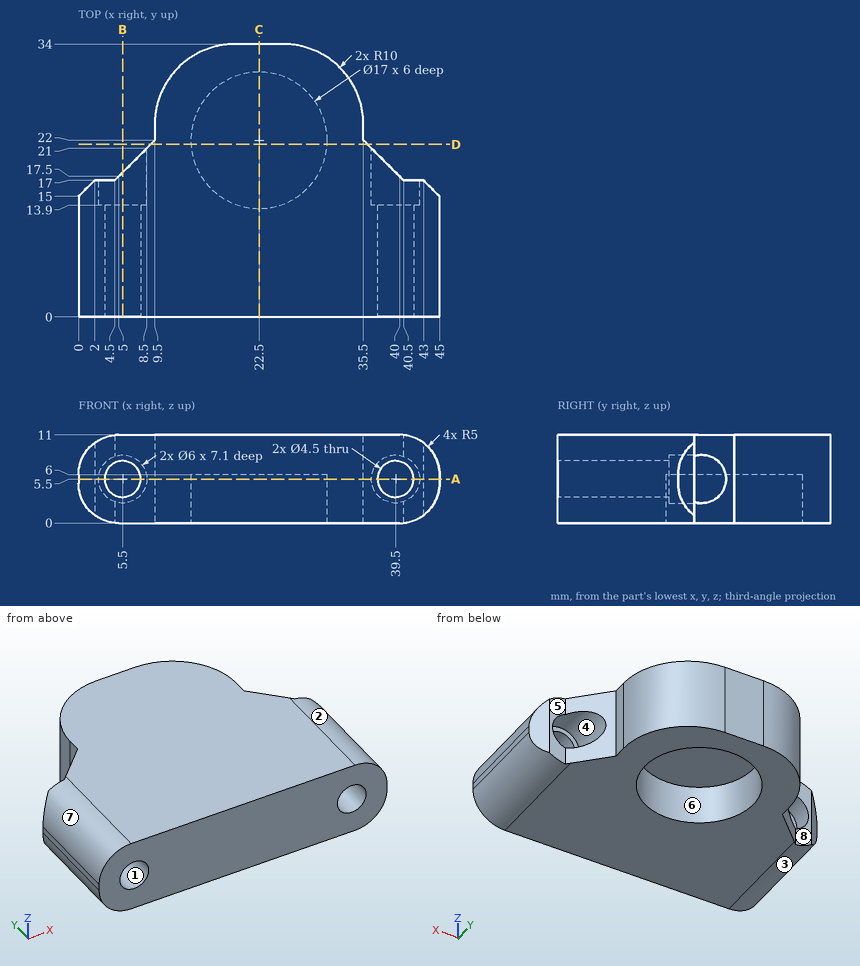
Study the drawing (mm; zero at the part's minimum x, y, z) and answer. A direction names the side the tool comes from. Give positions to 0.01 mm unless a question says otherwise; leave off trailing zeros. Write each loop counter-clockwise with the first axis right and the second up, starting at its lowest first coordinate (ties: lowest second). Pieces come first, ordered by that corner, then holes. Notation, with made-up numbers: (41, -25.75) -> (73, -25.75) arc R26 ccw to (73, 1.25) -> close; hole circle Ø11 at (4, -15). An arc over 180 degrees is marked (long way). Answer in a Markdown table with one row per item.
1) Section A-A on z = 5.5 is taken. Count the separate pieces of the cut face and the enclosed holes in it, plus the area to 3 significant figures.
Results list:
| item | result |
|---|---|
| separate pieces | 3 |
| enclosed holes | 1 |
| area | 780 mm^2 |
2) Each of these flat-tipped pins is pushed along its axis until it touches: pin 1 Ø5 at (x, y) = (26.5, 23) entering from -Z; pin 2 Ø5 at (x, z) = (39.5, 5.5) entering from -Y; pin 3 Ø0.8 at (x, z) = (41.5, 6.5) entering from +Y; pin 4 Ø3 at (x, z) = (40, 5.5) entering from +Y. Where does it stop, or does it pass through?
Results list:
| item | result |
|---|---|
| pin 1 | z = 6 |
| pin 2 | y = 0 |
| pin 3 | y = 13.9 |
| pin 4 | through |
3) Section C-C on x = 22.5 is taken. Give the vertices of the cut face in (y, z).
Results list:
| item | result |
|---|---|
| outline | (0, 0) -> (13.5, 0) -> (13.5, 6) -> (30.5, 6) -> (30.5, 0) -> (34, 0) -> (34, 11) -> (0, 11) -> close |
4) Section D-D on y = 21.5 is taken. Give the vertices of the cut face in (x, z).
Results list:
| item | result |
|---|---|
| outline | (9, 0) -> (14.01, 0) -> (14.01, 6) -> (30.99, 6) -> (30.99, 0) -> (36, 0) -> (36, 11) -> (9, 11) -> close |
5) Section B-B on x = 5.5 is taken. Give the vertices of the cut face in (y, z), plus the area to 3 significant figures.
Results list:
| item | result |
|---|---|
| outline | (0, 0) -> (18, 0) -> (18, 2.5) -> (13.9, 2.5) -> (13.9, 3.25) -> (0, 3.25) -> close; (0, 7.75) -> (13.9, 7.75) -> (13.9, 8.5) -> (18, 8.5) -> (18, 11) -> (0, 11) -> close |
| area | 111 mm^2 |
6) Determine the mould class of the marked faces 1, 2 and 3 for opening direction Z: released by +Z, released by -Z, zero draft, split by the parting line, or undercut.
Results list:
| item | result |
|---|---|
| face 1 | undercut |
| face 2 | released by +Z |
| face 3 | released by -Z |
7) Straight lines are drawn through the part: line 1 (Z direction, x = 39.5, y = 9); line 2 (Y direction, x = 22.5, z = 3.25); line 3 (X direction, y = 7, z = 4). For each, find the intervals that lie inside material, in ascending order. Write a range as [from, to].
Results list:
| item | result |
|---|---|
| line 1 | [0, 3.25], [7.75, 11] |
| line 2 | [0, 13.5], [30.5, 34] |
| line 3 | [0.1, 3.82], [7.18, 37.82], [41.18, 44.9] |
8) A tool of negligible diameter and unlimited length cuts with its end or side. For the marked faces 4, 5, 6, 7 and 8, from which of +Z, -Z, +X, -X, +Y, -Y can it reach the whole face along a straight path? Write none if from no direction.
Results list:
| item | result |
|---|---|
| face 4 | +Y |
| face 5 | +Z, -Z, +X, +Y |
| face 6 | -Z |
| face 7 | +Z, -X, +Y, -Y |
| face 8 | +Z, -Z, -X, +Y |
